Part model, mm, in its own coordinate system. Give positions to 0.01 mm unless a question says otherwise; leave off trailing zeros. Write each loop counter-clockwise with the first axis right and the second up, starting at its lowest first coordinate (ties: lowest second). Pieces come first, ordered by that corner, then holes.
```python
from build123d import *

# Parameters (mm, degrees)
SKETCH1_R           = 2.5
BOSS_EXTRUDE1_DEPTH = 4.75
SKETCH2_W           = 10
SKETCH2_H           = 4.75
SKETCH2_W_2         = 4.75
SKETCH2_H_2         = 10
CUT_EXTRUDE1_DEPTH  = 134.927452376
SKETCH3_R           = 1.5
CUT_EXTRUDE2_DEPTH  = 134.927452376
CAVITY1_OUTLINE_R   = 1.5
CAVITY1_DEPTH       = 4.75


# Read off the part's stored shape, not the designer's step: Cavity1
with BuildPart() as part:
    # Sketch1 → Boss-Extrude1 (new body)
    with BuildSketch(Plane.XY):
        with BuildLine():
            Line((-9.685424338, 2.488484559), (5.386220056, 61.148792841))
            ThreePointArc((5.386220056, 61.148792841), (15.733633721, 76.897010412), (33.561388608, 83))
            Line((33.561388608, 83), (105, 83))
            Line((105, 83), (105, 0))
            Line((105, 0), (-10.324792855, 0))
            Line((-10.324792855, 0), (-9.685424338, 2.488484559))
        make_face()
        with Locations((33.561388608, 53.909722104)):
            Circle(SKETCH1_R, mode=Mode.SUBTRACT)
    extrude(amount=BOSS_EXTRUDE1_DEPTH)

    # Sketch2 → Cut-Extrude1 (cut, through all)
    with BuildSketch(Plane.XY.offset(4.75)):
        with Locations((15, 2.375)):
            Rectangle(SKETCH2_W, SKETCH2_H)
        with Locations((57.5, 2.375)):
            Rectangle(SKETCH2_W, SKETCH2_H)
        with Locations((100, 2.375)):
            Rectangle(SKETCH2_W, SKETCH2_H)
        with Locations((102.625, 19.75)):
            Rectangle(SKETCH2_W_2, SKETCH2_H_2)
        with Locations((12.375, 19.75)):
            Rectangle(SKETCH2_W_2, SKETCH2_H_2)
    extrude(amount=-CUT_EXTRUDE1_DEPTH, mode=Mode.SUBTRACT)

    # Sketch3 → Cut-Extrude2 (cut, through all)
    with BuildSketch(Plane.XY.offset(4.75)):
        with Locations((50, 78)):
            Circle(SKETCH3_R)
        with Locations((100, 78)):
            Circle(SKETCH3_R)
    extrude(amount=-CUT_EXTRUDE2_DEPTH, mode=Mode.SUBTRACT)

    # Cavity1 outline → Cavity1 (cut)
    with BuildSketch(Plane.XY):
        with Locations((8.414860226, 52.844005614)):
            Circle(CAVITY1_OUTLINE_R)
    extrude(amount=CAVITY1_DEPTH, mode=Mode.SUBTRACT)


solid = part.part
```
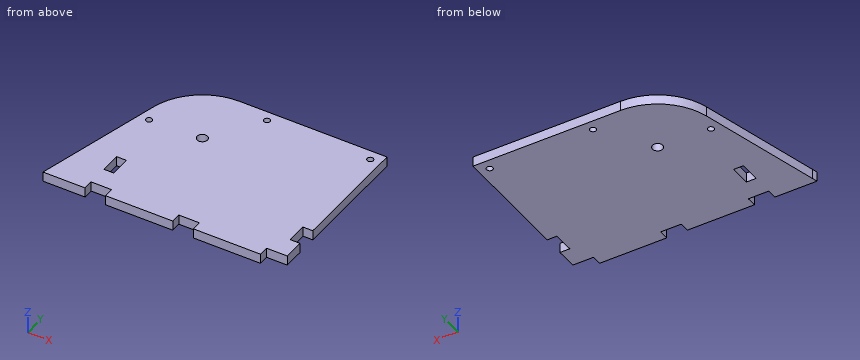
1) Saw through at B-B, the plane z = 1.45. Write the cut outline in (x, y).
Answers follow:
outline: (-10.32, 0) - (10, 0) - (10, 4.75) - (20, 4.75) - (20, 0) - (52.5, 0) - (52.5, 4.75) - (62.5, 4.75) - (62.5, 0) - (95, 0) - (95, 4.75) - (105, 4.75) - (105, 14.75) - (100.25, 14.75) - (100.25, 24.75) - (105, 24.75) - (105, 83) - (33.56, 83) arc R29.09 ccw to (5.39, 61.15) - close; hole circle Ø3 at (8.41, 52.84); hole (10, 14.75) - (14.75, 14.75) - (14.75, 24.75) - (10, 24.75) - close; hole circle Ø5 at (33.56, 53.91); hole circle Ø3 at (50, 78); hole circle Ø3 at (100, 78)
2) Saw through at C-C, the plane y = 21. Write the cut outline in (x, z), then the cut area to 3 significant figures.
Answers follow:
outline: (-4.93, 0) - (10, 0) - (10, 4.75) - (-4.93, 4.75) - close; (14.75, 0) - (100.25, 0) - (100.25, 4.75) - (14.75, 4.75) - close
area: 477 mm2
3) Saw through at D-D, the plane y = 78. Write the cut outline in (x, z), then the cut area to 3 significant figures.
Answers follow:
outline: (17.25, 0) - (48.5, 0) - (48.5, 4.75) - (17.25, 4.75) - close; (51.5, 0) - (98.5, 0) - (98.5, 4.75) - (51.5, 4.75) - close; (101.5, 0) - (105, 0) - (105, 4.75) - (101.5, 4.75) - close
area: 388 mm2
4) Saw through at A-A, the plane x = 50. Write the cut outline in (y, z).
Answers follow:
outline: (0, 0) - (76.5, 0) - (76.5, 4.75) - (0, 4.75) - close; (79.5, 0) - (83, 0) - (83, 4.75) - (79.5, 4.75) - close
5) Wall check: L1, parallel to Y at x = 100, z = 1.05; L2, parallel to X at y = 78, z = 2; L3, parallel to Y at x = 58.5, z = 3.15. Give the ranges that are in metal, low to high.
Answers follow:
L1: y = 4.75 to 76.5, 79.5 to 83
L2: x = 17.25 to 48.5, 51.5 to 98.5, 101.5 to 105
L3: y = 4.75 to 83
6) Pin check, flat tips, straight feed: pin 1 Ø1.4 at (y, z) = (1.5, 3.5) entering from +X; pin 2 Ø2.5 at (y, z) = (2, 2.5) entering from -X; pin 3 Ø2.5 at (x, y) = (50, 78) entering from -Z; pin 4 Ø1.4 at (x, z) = (13, 2.5) entering from +Y. Stop position of each tip, or through.
Answers follow:
pin 1: stops at x = 95
pin 2: stops at x = -10.13
pin 3: passes through
pin 4: stops at y = 75.16
